Study the drawing (mm; zero at the part's minimum x, y, z) and answer. A direction names the side the tool comes from. Give positions to 0.01 mm unless a question says otherwise; leave off trailing zeros. Order: outer loops, then holes, each group sorted by start corner. A loop starts at its lowest first (then second) coordinate and runs counter-clockwise, first axis right, second up.
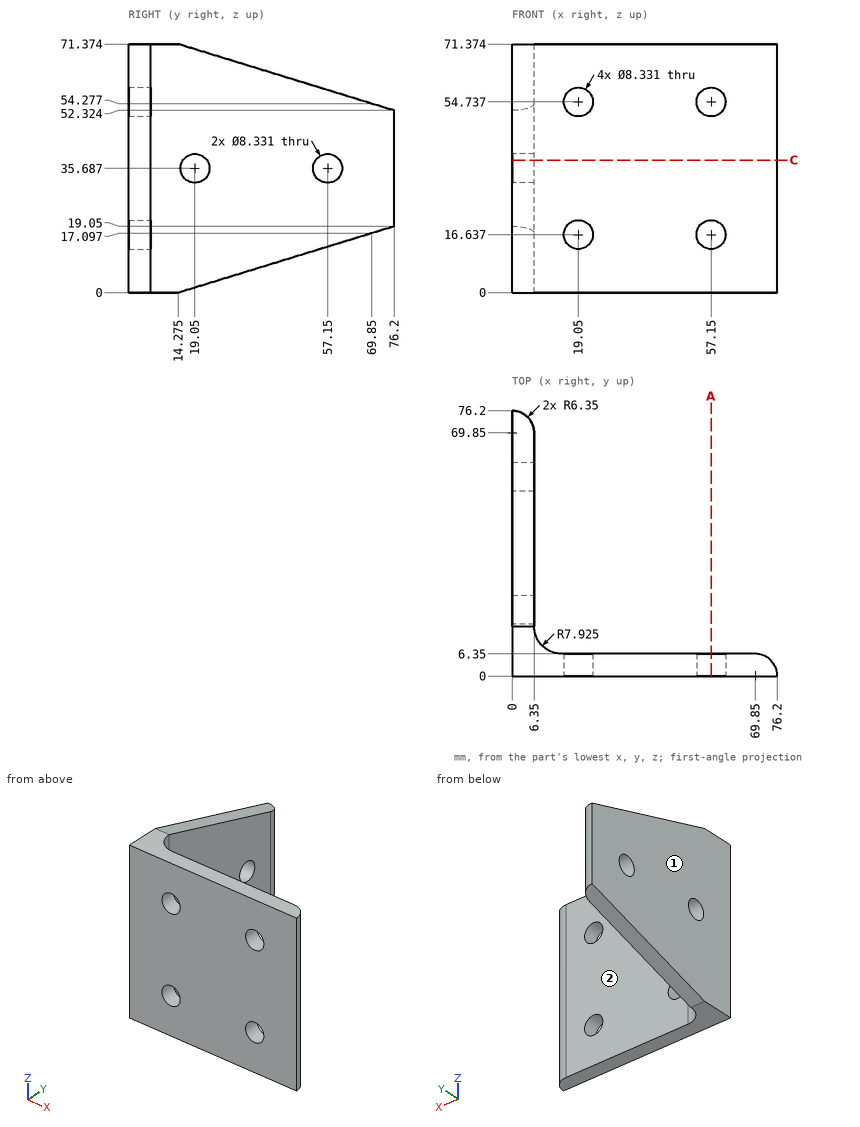
1) Straight lines are drawn through the part: probe 1 along Z at (x, y) = (57.15, 2.75); probe 2 along Y at (x, z) = (60.5, 40). For each, find the intervals that lie inside material, in ascending order.
Geometry says:
probe 1: z = 0 to 12.47, 20.8 to 50.57, 58.9 to 71.37
probe 2: y = 0 to 6.35
2) Given P1, Ø9.5, axis at x = 19.05, z = 16.637, coming from the +Y side; P2, Ø12, axis at x = 21, z = 39, coming from the +Y side, each flat-ended and moving along its own axis, determine where each tip first touches the part or whether it passes through.
Geometry says:
P1: stops at y = 6.35
P2: stops at y = 6.35
3) Find section C-C (z = 38). Count the separate pieces of the cut face and the enclosed holes in it.
Geometry says:
separate pieces: 3
enclosed holes: 0
4) Find section A-A (x = 57.15). Write down the section's boundary in (y, z).
Geometry says:
outline: (0, 0) - (6.35, 0) - (6.35, 12.47) - (0, 12.47) - close; (0, 20.8) - (6.35, 20.8) - (6.35, 50.57) - (0, 50.57) - close; (0, 58.9) - (6.35, 58.9) - (6.35, 71.37) - (0, 71.37) - close
5) A tool of negligible diameter and unlimited length cuts with its end or side. For the marked faces 1 and 2, from which of +Z, -Z, +X, -X, +Y, -Y can it reach the whole face along a straight path? Write none if from no direction.
Geometry says:
face 1: +Z, -Z, -X, +Y, -Y
face 2: +Z, -Z, +X, +Y
